Check sheet for the modelled part. Datum: model origin and axes. Units: mm. Face numbers are marked on the shaded views. A direction names the side the tool comes from. Coordinates: 2 decimals unless noted, no trailing zeros. Loops run counter-clockwise (first coordinate to the right, second up) from the corner with the lowest first, then second, coordinate; pieces in that order, holes last. Notation, with made-up numbers: M 11.5,-27.75 L 17.5,-27.75 A34 cw 17.5,2.25 Z; hole C -11.75,39.25 d1. An arc over 180 degrees is marked long. Answer as CSV lines item,"result". Start each with the question number.
from build123d import *

# Parameters (mm, degrees)
SZKIC1_R                    = 2
DODANIE_WYCI_GNI_CIE1_DEPTH = 2.9
SZKIC2_R                    = 3.5
SZKIC2_R_2                  = 2
DODANIE_WYCI_GNI_CIE2_DEPTH = 5


with BuildPart() as part:
    # Szkic1 → Dodanie-wyciągnięcie1 (new body)
    with BuildSketch(Plane.XY):
        Polygon((-4.041451884, 0), (-2.020725942, -3.5), (2.020725942, -3.5), (4.041451884, 0), (2.020725942, 3.5), (-2.020725942, 3.5), align=None)
        Circle(SZKIC1_R, mode=Mode.SUBTRACT)
    extrude(amount=DODANIE_WYCI_GNI_CIE1_DEPTH)

    # Szkic2 → Dodanie-wyciągnięcie2 (add)
    with BuildSketch(Plane.XY):
        Circle(SZKIC2_R)
        Circle(SZKIC2_R_2, mode=Mode.SUBTRACT)
    extrude(amount=DODANIE_WYCI_GNI_CIE2_DEPTH)

    # Szkic3 → Wycięcie-obrót1 (revolve, cut)
    with BuildSketch(Plane(origin=(0, 0, 0), x_dir=(1, 0, 0), z_dir=(0, 1, 0))):
        with BuildLine():
            Line((-4.041451884, 0), (-4.041451884, -0.441451884))
            ThreePointArc((-4.041451884, -0.441451884), (-3.912153621, -0.129298263), (-3.6, 0))
            Line((-3.6, 0), (-4.041451884, 0))
        make_face()
        with BuildLine():
            ThreePointArc((-3.6, -2.9), (-3.912153621, -2.770701737), (-4.041451884, -2.458548116))
            Line((-4.041451884, -2.458548116), (-4.041451884, -2.9))
            Line((-4.041451884, -2.9), (-3.6, -2.9))
        make_face()
        with BuildLine():
            Line((-3.5, -5), (-2.7, -5))
            ThreePointArc((-2.7, -5), (-3.265685425, -4.765685425), (-3.5, -4.2))
            Line((-3.5, -4.2), (-3.5, -5))
        make_face()
    revolve(axis=Axis((0, 0, -1.701574894), (0, 0, 1)), mode=Mode.SUBTRACT)


solid = part.part
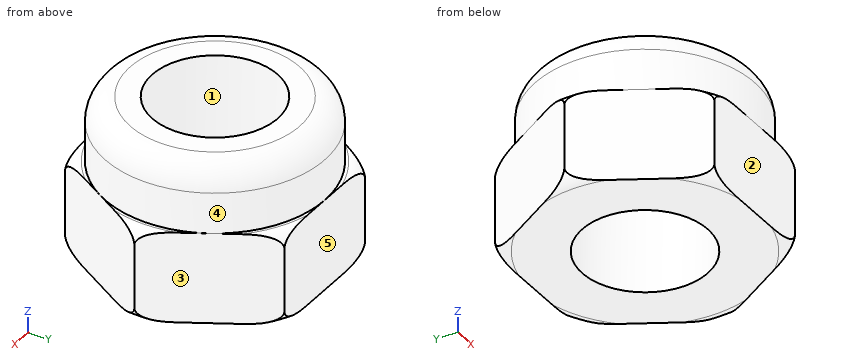
Item 1: Release check for a two-part mould opening along Y. For the marked faces 1, 2 and 3 record: released by +Y, released by -Y, zero draft, split by the parting line, or undercut.
Item 2: Sectioned sample at B-B, the plane z = 3. Record the boundary of the cut face in (x, y).
Item 3: Sectioned sample at A-A, the plane z = 1.35. Record the boundary of the cut face in (x, y), and give its area (3 significant figures).
Item 4: Go/stop test with flat-tipped pins: pin 1 (0.5 mm diameter, centred on x = -1, y = 3, fed in from +Z); pin 2 (1 mm diameter, centred on x = -3, z = 0.5, fed in from +Y). Record where each tip stops, or that it passes through.
Item 5: Set-up check for the marked faces 4 and 5: record each of +Z, -Z, +X, -X, +Y, -Y from which the full face is reachable in a straight line by a thin tool's end or side.
Item 6: Material ranges on line 1 (Y direction, x = 0, z = 2.2); line 2 (X direction, y = 0.5, z = 1.05); line 3 (Y direction, x = -1.5, z = 3.65), recorded low to high. Write a range as from..to.
Reply:
1,face 1,"undercut"
1,face 2,"released by -Y"
1,face 3,"released by +Y"
2,outline,"C 0,0 d7; hole C 0,0 d4"
3,outline,"M -4.04,0 L -2.02,-3.5 L 2.02,-3.5 L 4.04,0 L 2.02,3.5 L -2.02,3.5 Z; hole C 0,0 d4"
3,area,"29.9 mm²"
4,pin 1,"z = 4.97"
4,pin 2,"y = 2.67"
5,face 4,"+Z"
5,face 5,"+Z, -Z, +X, -X, +Y"
6,line 1,"-3.5..-2, 2..3.5"
6,line 2,"-3.75..-1.94, 1.94..3.75"
6,line 3,"-3.16..-1.32, 1.32..3.16"
